from build123d import *

# Parameters (mm, degrees)
SKETCH1_W           = 29.513896991
SKETCH1_H           = 12.7
SKETCH1_R           = 4.445
BOSS_EXTRUDE1_DEPTH = 15.875
SKETCH2_R           = 2.032
CUT_EXTRUDE1_DEPTH  = 12.7


with BuildPart() as part:
    # Sketch1 → Boss-Extrude1 (new body)
    with BuildSketch(Plane(origin=(0, 0, 0), x_dir=(1, 0, 0), z_dir=(0, 1, 0))):
        with Locations((14.756948496, 6.35)):
            Rectangle(SKETCH1_W, SKETCH1_H)
        with Locations((14.756948496, 7.14375)):
            Circle(SKETCH1_R, mode=Mode.SUBTRACT)
    extrude(amount=BOSS_EXTRUDE1_DEPTH)

    # Sketch2 → Cut-Extrude1 (cut)
    with BuildSketch(Plane(origin=(0, 0, -12.7), x_dir=(-1, 0, 0), z_dir=(0, 0, -1))):
        with Locations((-5.155974248, 7.9375)):
            Circle(SKETCH2_R)
        with Locations((-24.357922743, 7.9375)):
            Circle(SKETCH2_R)
    extrude(amount=-CUT_EXTRUDE1_DEPTH, mode=Mode.SUBTRACT)


solid = part.part
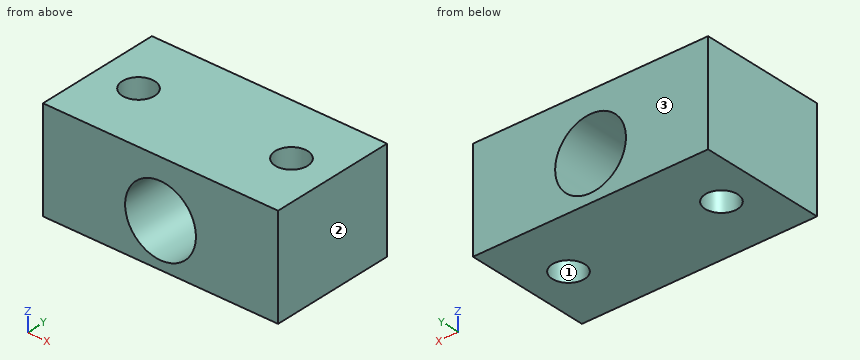
Could you check a few things on this model? Use its own coordinates, in mm. Face numbers are marked on the shaded views. Give positions to 0.01 mm unless a question says otherwise; leave off trailing zeros. Order: outer loops, then holes, each group sorted by start corner. A loop starts at its lowest first (then second) coordinate and runs counter-clockwise, first axis right, second up.
Item 1: If we section it at B-B, the plane z = -4.5: Write out the boundary of the cut face in (x, y) (1 decimal), plus the area to 3 significant figures.
Item 2: If we section it at D-D, the plane z = -7.5: Write out the boundary of the cut face in (x, y) (1 decimal).
Item 3: If we section it at A-A, the plane y = 8.5: Write out the boundary of the cut face in (x, z) (3 decimals).
Item 4: I need wall thicknesses on line 1 (X direction, y = 6.5, z = -6.75); line 2 (Z direction, x = 15, y = 8.5); line 3 (X direction, y = 7.25, z = -2.5). Which ranges of each line are inside material? Lowest first, please.
Item 5: If we mould it in two halves opening along X, with no side actions, what happens to the marked faces 1, 2 and 3? For each: pulls with the +X half, pulls with the -X half, needs draft (parallel to the pull), parting line crosses it, or undercut.
Item 6: If we section it at C-C, the plane x = 14.25: Write out the boundary of the cut face in (y, z) (3 decimals).
Values:
1. outline: (0, 0) - (11.2, 0) - (11.2, 15.9) - (0, 15.9) - close; (18.3, 0) - (29.5, 0) - (29.5, 15.9) - (18.3, 15.9) - close; hole circle Ø4.1 at (5.2, 7.9); hole circle Ø4.1 at (24.4, 7.9)
1. area: 329 mm2
2. outline: (0, 0) - (10.3, 0) - (10.3, 15.9) - (0, 15.9) - close; (19.2, 0) - (29.5, 0) - (29.5, 15.9) - (19.2, 15.9) - close; hole circle Ø4.1 at (5.2, 7.9); hole circle Ø4.1 at (24.4, 7.9)
3. outline: (0, -12.7) - (3.203, -12.7) - (3.203, 0) - (0, 0) - close; (7.109, -12.7) - (22.405, -12.7) - (22.405, 0) - (7.109, 0) - close; (26.311, -12.7) - (29.514, -12.7) - (29.514, 0) - (26.311, 0) - close; hole circle Ø8.89 at (14.757, -7.144)
4. line 1: x = 0 to 3.72, 6.59 to 10.33, 19.18 to 22.92, 25.79 to 29.51
4. line 2: z = -12.7 to -11.58, -2.71 to 0
4. line 3: x = 0 to 3.24, 7.07 to 22.45, 26.27 to 29.51
5. face 1: undercut
5. face 2: pulls with the +X half
5. face 3: needs draft
6. outline: (0, -12.7) - (15.875, -12.7) - (15.875, -11.56) - (0, -11.56) - close; (0, -2.728) - (15.875, -2.728) - (15.875, 0) - (0, 0) - close
